from build123d import *

# Parameters (mm, degrees)
SKETCH1_R           = 30
SKETCH1_R_2         = 15
BOSS_EXTRUDE1_DEPTH = 25
BOSS_EXTRUDE2_DEPTH = 5
SKETCH3_R           = 6
BOSS_EXTRUDE4_DEPTH = 9


with BuildPart() as part:
    # Sketch1 → Boss-Extrude1 (new body, symmetric)
    with BuildSketch(Plane.XY):
        Circle(SKETCH1_R)
        Circle(SKETCH1_R_2, mode=Mode.SUBTRACT)
    extrude(amount=BOSS_EXTRUDE1_DEPTH, both=True)

    # Sketch2 → Boss-Extrude2 (add, symmetric)
    with BuildSketch(Plane.XY):
        with BuildLine():
            Line((-3.948644693, 29.739001414), (-97.5, 17.317566762))
            Line((-97.5, 17.317566762), (-122.5, 17.317566762))
            Line((-122.5, 17.317566762), (-122.5, -12.682433238))
            Line((-122.5, -12.682433238), (-97.5, -12.682433238))
            Line((-97.5, -12.682433238), (-5.392030099, -29.511455596))
            ThreePointArc((-5.392030099, -29.511455596), (-29.99110227, 0.730605661), (-3.948644693, 29.739001414))
        make_face()
    extrude(amount=BOSS_EXTRUDE2_DEPTH, both=True)

    # Sketch3 → Boss-Extrude4 (add)
    with BuildSketch(Plane.XZ.offset(12.682433238)):
        with BuildLine():
            Line((-122.5, 5), (-97.5, 5))
            Line((-97.5, 5), (-97.5, 20))
            ThreePointArc((-97.5, 20), (-110, 32.5), (-122.5, 20))
            Line((-122.5, 20), (-122.5, 5))
        make_face()
        with Locations(Location((-110, 20, 0), (0, 0, 270))):  # turned: the seam where the file's is
            Circle(SKETCH3_R, mode=Mode.SUBTRACT)
    boss_extrude4 = extrude(amount=-BOSS_EXTRUDE4_DEPTH)

    # Mirror1: Boss-Extrude4 across plane
    add(boss_extrude4.mirror(Plane.ZX))


solid = part.part
Work out the finished part from the listing and answer in its coordinate system (mm). A direction names the side the tool comes from. Give positions to 0.01 mm unless a question says otherwise; leave off trailing zeros. Order: outer loops, then holes, each group sorted by start corner. A loop starts at its lowest first (then second) coordinate and runs counter-clockwise, first axis right, second up. Notation, with made-up numbers: (62, 34.25) -> (76, 34.25) arc R16 ccw to (76, 59.25) -> close; hole circle Ø11 at (39.5, 72.5). An arc over 180 degrees is marked (long way). One line per item, written item: value.
Item 1: A tool of negligible diameter and unlimited length cuts with its end or side. For faces 1 (the flat face through (6, 14, 25)), 2 (the flat face through (-97.5, -8, 12)), 3 (the flat face through (-110, -3.682, 13)), from which of +Z, -Z, +X, -X, +Y, -Y can it reach the whole face along a straight path? Write none if from no direction.
Answer sheet:
face 1: +Z, +X, +Y, -Y
face 2: +Z, +Y, -Y
face 3: +Z, -X
Item 2: Flat-ended cylindrical pins translate along their axes: P1, Ø10, axis at x = -25, z = 22.5, coming from the +Y side; P2, Ø8, axis at x = -25.5, y = 3.5, coming from the +Z side; P3, Ø19, axis at x = -110, z = 20, coming from the -Y side. Find the tip coordinate at first contact, or state that the pin passes through.
Answer sheet:
P1: y = 22.36
P2: z = 25
P3: y = -12.68
Item 3: Find section D-D, the plane z = -3.5. Give the vertices of the cut face in (x, y), plus the area to 3 significant figures.
Answer sheet:
outline: (-122.5, -12.68) -> (-97.5, -12.68) -> (-5.39, -29.51) arc R30 ccw (long way) to (-3.95, 29.74) -> (-97.5, 17.32) -> (-122.5, 17.32) -> close; hole circle Ø30 at (0, 0)
area: 5,880 mm²
Item 4: Find section C-C, the plane x = 0. Give the vertices of the cut face in (y, z).
Answer sheet:
outline: (-30, -25) -> (-15, -25) -> (-15, 25) -> (-30, 25) -> close; (15, -25) -> (30, -25) -> (30, 25) -> (15, 25) -> close
Item 5: Find section B-B, the plane y = 0. Give the vertices of the cut face in (x, z).
Answer sheet:
outline: (-122.5, -5) -> (-30, -5) -> (-30, -25) -> (-15, -25) -> (-15, 25) -> (-30, 25) -> (-30, 5) -> (-122.5, 5) -> close; (15, -25) -> (30, -25) -> (30, 25) -> (15, 25) -> close
Item 6: Find section A-A, the plane z = 7. Give the vertices of the cut face in (x, y).
Answer sheet:
outline: (-122.5, -12.68) -> (-97.5, -12.68) -> (-97.5, -3.68) -> (-122.5, -3.68) -> close; (-122.5, 3.68) -> (-97.5, 3.68) -> (-97.5, 12.68) -> (-122.5, 12.68) -> close; circle Ø60 at (0, 0); hole circle Ø30 at (0, 0)
Item 7: Determine the mould class of faces 4 (the flat face through (-110, -12.682, 10)), 5 (the cylindrical face through (-109.725, -8.245, 32.497)), 6 (the cylindrical face through (-14.985, 0.66, -0.35)) for opening direction Y: released by +Y, released by -Y, zero draft, split by the parting line, or undercut.
Answer sheet:
face 4: released by -Y
face 5: zero draft
face 6: undercut
Item 8: Straight lines are drawn through the part: probe 1 along Y at (x, z) = (0, 4.5); probe 2 along X at (y, z) = (9, 20); probe 3 along X at (y, z) = (-6, 20). For each, find the intervals that lie inside material, in ascending order.
Answer sheet:
probe 1: -30 to -15, 15 to 30
probe 2: -122.5 to -116, -104 to -97.5, -28.62 to -12, 12 to 28.62
probe 3: -122.5 to -116, -104 to -97.5, -29.39 to -13.75, 13.75 to 29.39
